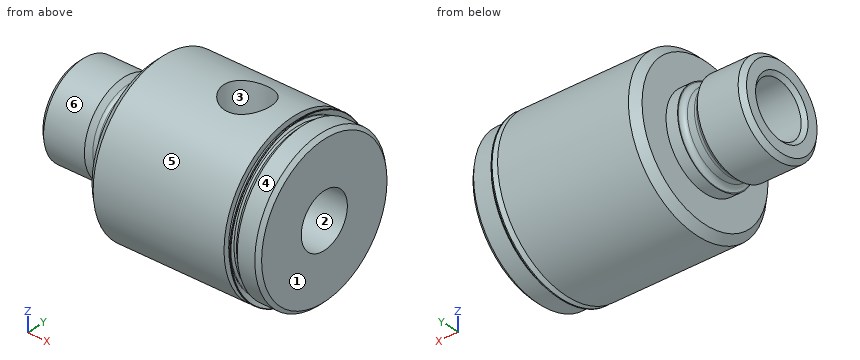
Autodesk Inventor part; units mm, degrees
ref_plane "dp1_XY" through (15.8496, 9.4932, 0) normal (0, 0, 1) x (1, 0, 0)
ref_plane "dp1_YZ" through (15.8496, 9.4932, 0) normal (1, 0, 0) x (0, 1, 0)
ref_plane "dp1_ZX" through (15.8496, 9.4932, 0) normal (0, 1, 0) x (0, 0, 1)
sketch "Sketch_2" plane through (0, 0, 0) normal (0, 0, 1) x (1, 0, 0)
  line L0 (15.8496, 0) -> (0, 0)
  line L1 (0, 0) -> (0, 8.589)
  line L2 (0, 8.589) -> (0.936, 9.525)
  line L3 (0.936, 9.525) -> (9.3565, 9.525)
  line L4 (9.3565, 9.525) -> (10.2956, 8.594)
  arc A0 (10.2956, 8.594) -> (11.0109, 8.2995) centre (11.0109, 9.3154) ccw
  line L5 (11.0109, 8.2995) -> (12.446, 8.2995)
  arc A1 (12.446, 8.2995) -> (13.462, 9.3155) centre (12.446, 9.3154) ccw
  line L6 (13.462, 9.3155) -> (13.462, 9.4932)
  line L7 (13.462, 9.4932) -> (15.8496, 9.4932)
  line L8 (15.8496, 9.4932) -> (15.8496, 0)
  line L9 (15.8496, 0) -> (0, 0)
revolve "Revolution1" add sketch "Sketch_2" angle 360 about axis through (15.8496, 0, 0) along (1, 0, 0)
thread "Thread1"
sketch "Sketch_3" plane through (0, 0, 0) normal (0, 0, 1) x (1, 0, 0)
  line L0 (50.8, 0) -> (15.8496, 0)
  line L1 (15.8496, 0) -> (15.8496, 15.3226)
  line L2 (15.8496, 15.3226) -> (17.3736, 16.8466)
  line L3 (17.3736, 16.8466) -> (44.3865, 16.8466)
  line L4 (44.3865, 16.8466) -> (44.3865, 15.0051)
  line L5 (44.3865, 15.0051) -> (45.4025, 15.0051)
  line L6 (45.4025, 15.0051) -> (46.4185, 16.021)
  line L7 (46.4185, 16.021) -> (50.038, 16.021)
  line L8 (50.038, 16.021) -> (50.8, 15.2591)
  line L9 (50.8, 15.2591) -> (50.8, 0)
  line L10 (50.8, 0) -> (15.8496, 0)
revolve "Revolution2" add sketch "Sketch_3" angle 360 about axis through (50.8, 0, 0) along (1, 0, 0)
sketch "Sketch3" plane through (0, 0, 0) normal (-1, 0, 0) x (0, 0, 1)
  point P0 (0, 0)
hole "Hole1" at (0, 0, 0) direction (1, 0, 0) diameter 11.2268 depth 50.8 countersink diameter 12.7508 countersink angle 90
sketch "Sketch_40" plane through (0, 0, 0) normal (0, 1, 0) x (-1, 0, 0)
  line L0 (-34.925, 16.8466) -> (-34.925, 0)
  line L1 (-34.925, 0) -> (-38.1, 0)
  line L2 (-38.1, 0) -> (-38.1, 5.9544)
  line L3 (-38.1, 5.9544) -> (-39.4671, 7.3216)
  line L4 (-39.4671, 7.3216) -> (-39.7645, 16.8466)
  line L5 (-39.7645, 16.8466) -> (-34.925, 16.8466)
  line L6 (-34.925, 16.8466) -> (-34.925, 0)
revolve "Revolution3" cut sketch "Sketch_40" angle 360 about axis through (34.925, 0, 16.8466) along (0, 0, 1)
thread "Thread2"
sketch "Sketch_47" plane through (0, 0, 0) normal (0, 0, 1) x (1, 0, 0)
  line L0 (45.4025, 0) -> (44.3865, 0)
  line L1 (44.3865, 15.7133) -> (44.3865, 14.7511)
  line L2 (44.3865, 14.7511) -> (45.4025, 14.7511)
  line L3 (45.4025, 14.7511) -> (45.4025, 15.0051)
  line L4 (45.4025, 15.0051) -> (44.8945, 15.0051)
  line L5 (44.8945, 15.0051) -> (44.5199, 15.3797)
  arc A0 (44.5199, 15.5593) -> (44.5199, 15.3797) centre (44.6097, 15.4695) ccw
  line L6 (44.5199, 15.5593) -> (45.723, 16.7624)
  line L7 (45.723, 16.7624) -> (45.723, 16.8466)
  line L8 (45.723, 16.8466) -> (45.5198, 16.8466)
  line L9 (45.5198, 16.8466) -> (44.3865, 15.7133)
revolve "Revolution4" add sketch "Sketch_47" angle 360 about axis through (45.4025, 0, 0) along (1, 0, 0)
ref_plane "dp1_XY" through (15.8496, 9.4932, 0) normal (0, 0, 1) x (1, 0, 0)
ref_plane "dp1_YZ" through (15.8496, 9.4932, 0) normal (1, 0, 0) x (0, 1, 0)
ref_plane "dp1_ZX" through (15.8496, 9.4932, 0) normal (0, 1, 0) x (0, 0, 1)
ref_plane "dp2_XY" through (15.8496, -9.4932, 0) normal (0, 0, 1) x (1, 0, 0)
ref_plane "dp2_YZ" through (15.8496, -9.4932, 0) normal (1, 0, 0) x (0, 1, 0)
ref_plane "dp2_ZX" through (15.8496, -9.4932, 0) normal (0, 1, 0) x (0, 0, 1)
ref_plane "hh_XY" through (0, 9.525, 0) normal (0, 0, 1) x (1, 0, 0)
ref_plane "hh_YZ" through (0, 9.525, 0) normal (1, 0, 0) x (0, 1, 0)
ref_plane "hh_ZX" through (0, 9.525, 0) normal (0, 1, 0) x (0, 0, 1)
ref_plane "port_XY" through (34.925, 0, 0) normal (0, 0, 1) x (1, 0, 0)
ref_plane "port_YZ" through (34.925, 0, 0) normal (1, 0, 0) x (0, 1, 0)
ref_plane "port_ZX" through (34.925, 0, 0) normal (0, 1, 0) x (0, 0, 1)
ref_plane "rod_guide_XY" through (0, 0, 0) normal (1, 0, 0) x (0, 0, -1)
ref_plane "rod_guide_YZ" through (0, 0, 0) normal (0, 0, -1) x (0, 1, 0)
ref_plane "rod_guide_ZX" through (0, 0, 0) normal (0, 1, 0) x (1, 0, 0)
ref_plane "s1_XY" through (13.462, 0, 0) normal (0, 0, 1) x (1, 0, 0)
ref_plane "s1_YZ" through (13.462, 0, 0) normal (1, 0, 0) x (0, 1, 0)
ref_plane "s1_ZX" through (13.462, 0, 0) normal (0, 1, 0) x (0, 0, 1)
ref_plane "s2_XY" through (15.8496, 0, 0) normal (0, 0, 1) x (1, 0, 0)
ref_plane "s2_YZ" through (15.8496, 0, 0) normal (1, 0, 0) x (0, 1, 0)
ref_plane "s2_ZX" through (15.8496, 0, 0) normal (0, 1, 0) x (0, 0, 1)
ref_plane "t1_XY" through (15.8496, 0, 0) normal (1, 0, 0) x (0, 0, -1)
ref_plane "t1_YZ" through (15.8496, 0, 0) normal (0, 0, -1) x (0, 1, 0)
ref_plane "t1_ZX" through (15.8496, 0, 0) normal (0, 1, 0) x (1, 0, 0)
ref_plane "t111_XY" through (15.8496, 0, 0) normal (1, 0, 0) x (0, 0, -1)
ref_plane "t111_YZ" through (15.8496, 0, 0) normal (0, 0, -1) x (0, 1, 0)
ref_plane "t111_ZX" through (15.8496, 0, 0) normal (0, 1, 0) x (1, 0, 0)
ref_plane "to_foot_bracket_XY" through (15.8496, 0, 0) normal (1, 0, 0) x (0, 0, -1)
ref_plane "to_foot_bracket_YZ" through (15.8496, 0, 0) normal (0, 0, -1) x (0, 1, 0)
ref_plane "to_foot_bracket_ZX" through (15.8496, 0, 0) normal (0, 1, 0) x (1, 0, 0)
ref_plane "to_nut_XY" through (13.462, 0, 0) normal (1, 0, 0) x (0, 0, -1)
ref_plane "to_nut_YZ" through (13.462, 0, 0) normal (0, 0, -1) x (0, 1, 0)
ref_plane "to_nut_ZX" through (13.462, 0, 0) normal (0, 1, 0) x (1, 0, 0)
ref_plane "to_rod_XY" through (0, 0, 0) normal (1, 0, 0) x (0, 0, -1)
ref_plane "to_rod_YZ" through (0, 0, 0) normal (0, 0, -1) x (0, 1, 0)
ref_plane "to_rod_ZX" through (0, 0, 0) normal (0, 1, 0) x (1, 0, 0)
ref_plane "to_screw_XY" through (34.925, 0, 0) normal (0, 1, 0) x (1, 0, 0)
ref_plane "to_screw_YZ" through (34.925, 0, 0) normal (1, 0, 0) x (0, 0, -1)
ref_plane "to_screw_ZX" through (34.925, 0, 0) normal (0, 0, -1) x (0, 1, 0)
ref_plane "to_trunnion_brackets_XY" through (0, 0, 0) normal (0, 1, 0) x (1, 0, 0)
ref_plane "to_trunnion_brackets_YZ" through (0, 0, 0) normal (1, 0, 0) x (0, 0, -1)
ref_plane "to_trunnion_brackets_ZX" through (0, 0, 0) normal (0, 0, -1) x (0, 1, 0)
ref_plane "to_trunnion_brackets1_XY" through (0, 0, 0) normal (0, 1, 0) x (1, 0, 0)
ref_plane "to_trunnion_brackets1_YZ" through (0, 0, 0) normal (1, 0, 0) x (0, 0, -1)
ref_plane "to_trunnion_brackets1_ZX" through (0, 0, 0) normal (0, 0, -1) x (0, 1, 0)
ref_plane "to_trunnion_brackets2_XY" through (0, 0, 0) normal (0, 1, 0) x (1, 0, 0)
ref_plane "to_trunnion_brackets2_YZ" through (0, 0, 0) normal (1, 0, 0) x (0, 0, -1)
ref_plane "to_trunnion_brackets2_ZX" through (0, 0, 0) normal (0, 0, -1) x (0, 1, 0)
ref_plane "to_tube_XY" through (45.4025, 0, 0) normal (1, 0, 0) x (0, 0, -1)
ref_plane "to_tube_YZ" through (45.4025, 0, 0) normal (0, 0, -1) x (0, 1, 0)
ref_plane "to_tube_ZX" through (45.4025, 0, 0) normal (0, 1, 0) x (1, 0, 0)
properties part number "12R000-0_rod_guide"
Read the model definition and answer for the solid it produces. Units are mm, in the model's axes. Face numbers are marked on the shaded views. A direction names the side the tool comes from. Coordinates: 2 decimals unless noted, no trailing zeros. Loops run counter-clockwise (first coordinate to the right, second up) from the corner with the lowest first, then second, coordinate; pieces in that order, holes last. Notation, with made-up numbers: (-6.5, 77.25) - (28.5, 77.25) arc R23 cw to (28.5, 89.25) - close; hole circle Ø7 at (23.5, 65.25). An arc over 180 degrees is marked (long way). Answer in a Markdown table with one row per item.
Q1. Straight lines are drawn through the part: line 1 along Z through (x, y) = (45, 4.5); line 2 along Z through (x, y) = (26, 0); line 3 along X through (y, z) = (-9.5, -11). For each, find the intervals that lie inside material, in ascending order. Write a range as [from, to].
Here are the results:
| item | result |
|---|---|
| line 1 | z = [-15.69, -15.4], [-14.31, -3.36], [3.36, 14.31], [15.4, 15.69] |
| line 2 | z = [-16.85, -5.61], [5.61, 16.85] |
| line 3 | x = [15.85, 50.8] |
Q2. Find section C-C on x = 47.5. Write down the section's boundary in (y, z), plus the area to 3 significant figures.
Here are the results:
| item | result |
|---|---|
| outline | circle Ø32.04 at (0, 0); hole circle Ø11.23 at (0, 0) |
| area | 707 mm^2 |
Q3. Find section A-A on x = 7.5. Write down the section's boundary in (y, z) (3 decimals), plus the area to 3 significant figures.
Here are the results:
| item | result |
|---|---|
| outline | circle Ø19.05 at (0, 0); hole circle Ø11.227 at (0, 0) |
| area | 186 mm^2 |
Q4. The mould has two halves that part along X. Classify the marked faces 1, 2 and 3: pulls with the +X half, pulls with the -X half, needs draft (parallel to the pull), parting line crosses it, or undercut.
Here are the results:
| item | result |
|---|---|
| face 1 | pulls with the +X half |
| face 2 | needs draft |
| face 3 | undercut |
Q5. Find section B-B on y = -2.5. Count the separate pieces of the cut face and the enclosed holes in it, plus the area to 3 significant figures.
Here are the results:
| item | result |
|---|---|
| separate pieces | 3 |
| enclosed holes | 0 |
| area | 834 mm^2 |
Q6. For the marked faces 4, 5 and 6, determine the directions among +Z, -Z, +X, -X, +Y, -Y from which every point of the face is accessible in a straight line to the end or side of a thin tool.
Here are the results:
| item | result |
|---|---|
| face 4 | +X |
| face 5 | +X, -X |
| face 6 | -X |
Q7. Given P1, Ø1.5, axis at x = 11.5, y = 3, coming from the +Z side; P2, Ø12, axis at x = 16.5, z = -7, coming from the +Y side; P3, Ø5, axis at y = 12.5, z = -9, coming from the -X side, each flat-ended and moving along its own axis, determine where each tip first touches the part or whether it passes through.
Here are the results:
| item | result |
|---|---|
| P1 | stops at z = 7.99 |
| P2 | stops at y = 16.81 |
| P3 | stops at x = 15.85 |
